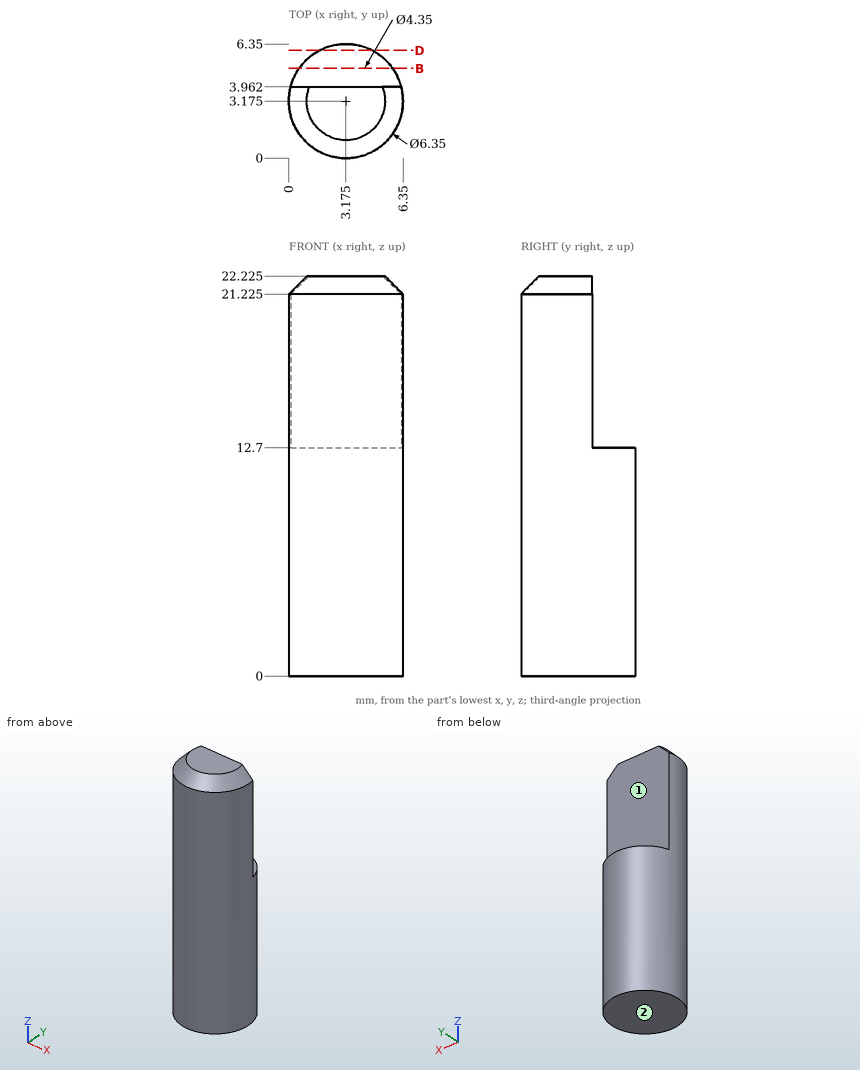
Geometry check sheet. Reference: drawing and pictorial views, mm from the part's lowest x, y, z. A direction names the side the tool comes from. Give positions to 0.01 mm unless a question says otherwise; leave off trailing zeros. Order: outer loops, then holes, each group sorted by start corner. A loop starts at its lowest first (then second) coordinate and runs counter-clockwise, first axis right, second up. Notation, with made-up numbers: (-0.5, 8.25) - (37.5, 8.25) arc R16 ccw to (37.5, 37.25) - close; hole circle Ø9 at (63.5, 58). An arc over 180 degrees is marked (long way). Answer as CSV lines item,"result".
1. Section check B-B (y = 5). Record the boundary of the cut face in (x, z).
Result sheet:
outline,"(0.58, 0) - (5.77, 0) - (5.77, 12.7) - (0.58, 12.7) - close"
2. Go/stop test with flat-tipped pins: P1, Ø2.5, axis at x = 4.5, y = 5.5, coming from the +Z side; P2, Ø1.5, axis at x = 5.5, z = 12.5, coming from the +Y side; P3, Ø3, axis at x = 3, z = 18.5, coming from the +Y side. Record where each tip stops, or that it passes through.
Result sheet:
P1,"z = 12.7"
P2,"y = 5.93"
P3,"y = 3.96"
3. Scan lines: probe 1 along Y at (x, z) = (3, 20.75) (1 decimal); probe 2 along Y at (x, z) = (3.25, 7); probe 3 along Z at (x, y) = (2, 4). Record each from-to range of solid material in increasing order. Write a range as from..to.
Result sheet:
probe 1,"0..4"
probe 2,"0..6.35"
probe 3,"0..12.7"
4. Section check D-D (y = 6). Record the boundary of the cut face in (x, z).
Result sheet:
outline,"(1.73, 0) - (4.62, 0) - (4.62, 12.7) - (1.73, 12.7) - close"
5. Tool access check on the marked faces 1 and 2. Record the directions out of +Z, -Z, +X, -X, +Y, -Y that give a thin tool (end or side, any length) a straight path to the whole face; none if there is none.
Result sheet:
face 1,"+Z, +X, -X, +Y"
face 2,"-Z, +X, -X, +Y, -Y"
